Part print with two shaded views. Sizes in mm from the minimum x, y, z corner. Coordinates: 2 decimals unless noted, no trailing zeros. Loops run counter-clockwise (first coordinate to the right, second up) from the corner with the lowest first, then second, coordinate; pieces in that order, holes last.
(1) Slice it at A-A (y = 76.2). Give the cut face in (x, z), and give its area (3 significant figures).
(2) Flat gauge pins, fed straight in: P1, Ø4, axis at x = 56, y = 30, coming from the +Z side; P2, Ø8, axis at x = 93.5, z = 10.5, coming from the +Y side; P3, Ø8, axis at y = 65.5, z = 56, coming from the -X side. Where does each tip first touch, or does it go through?
(3) Slice it at C-C (z = 30). Give the cut face in (x, y).
(4) Two-plate mould, pull along Y, no slides. Class the marked faces 1, 2 and 3: pulls with the +Y half, pulls with the -Y half, needs draft (parallel to the pull), parting line crosses it, or undercut.
(5) Wall check: L1, parallel to Y at x = 74.5, z = 32; L2, parallel to X at y = 76, z = 26; L3, parallel to Y at x = 39, z = 46. Give the ranges that are in metal, low to high.
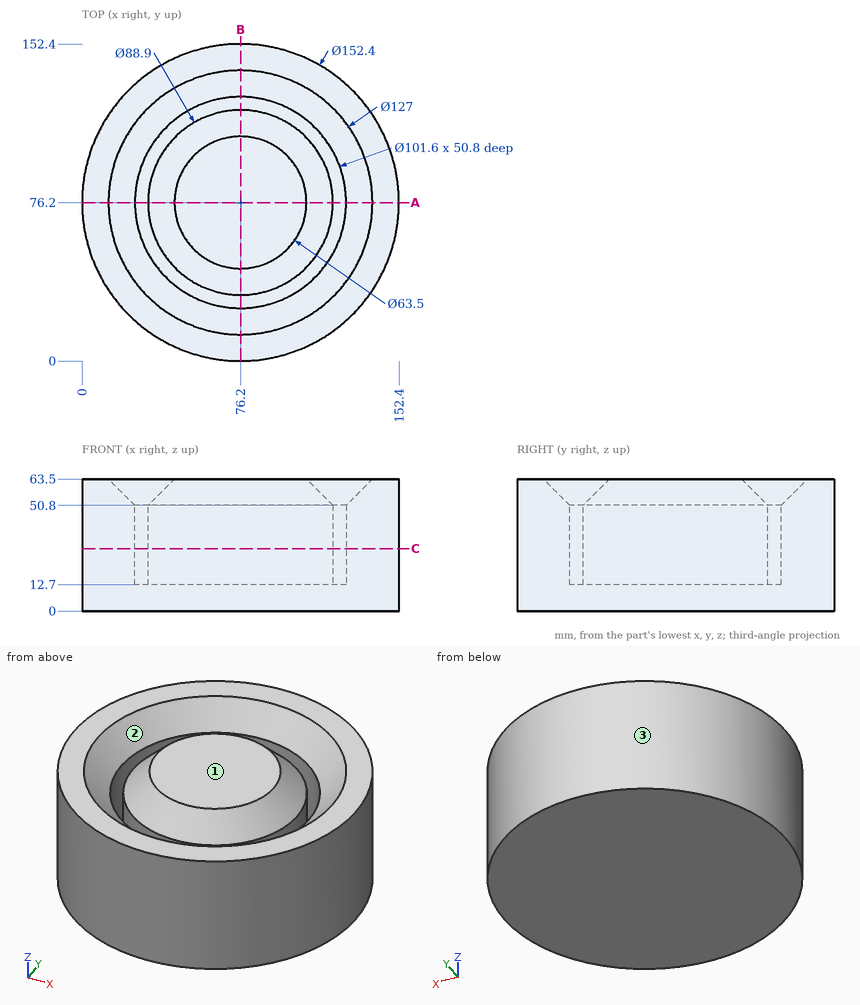
Response values:
1. outline: (0, 0) - (152.4, 0) - (152.4, 63.5) - (139.7, 63.5) - (127, 50.8) - (127, 12.7) - (120.65, 12.7) - (120.65, 50.8) - (107.95, 63.5) - (44.45, 63.5) - (31.75, 50.8) - (31.75, 12.7) - (25.4, 12.7) - (25.4, 50.8) - (12.7, 63.5) - (0, 63.5) - close
1. area: 8,710 mm2
2. P1: stops at z = 52.42
2. P2: stops at y = 151.23
2. P3: stops at x = 0.3
3. outline: circle Ø152.4 at (76.2, 76.2); circle Ø88.9 at (76.2, 76.2); hole circle Ø101.6 at (76.2, 76.2)
4. face 1: needs draft
4. face 2: undercut
4. face 3: parting line crosses it
5. L1: y = 0.02 to 25.43, 31.78 to 120.62, 126.97 to 152.38
5. L2: x = 0 to 25.4, 31.75 to 120.65, 127 to 152.4
5. L3: y = 9.7 to 41.61, 51.87 to 100.53, 110.79 to 142.7
